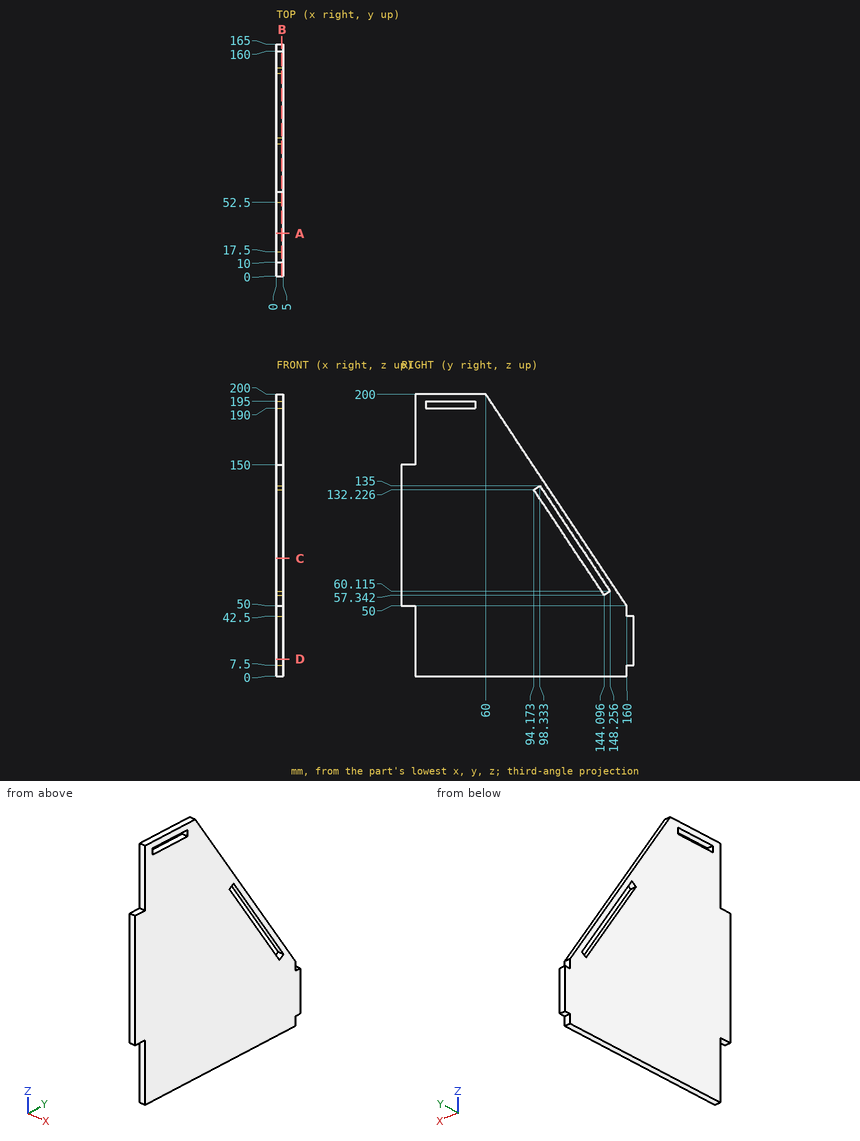
Study the drawing (mm; zero at the part's minimum x, y, z) and answer. Coordinates: 2 decimals unless noted, no trailing zeros. Order: outer loops, then holes, each group sorted by start corner. A loop starts at its lowest first (then second) coordinate and runs counter-clockwise, first axis right, second up. Notation, with made-up numbers: M -29,37.25 L -13,37.25 A25 ccw -13,55.25 Z; hole C -3,13 d9. An arc over 180 degrees is marked long. Use CSV: the item, a comma, the result in double quotes.
Q1. Section D-D (z = 12) is taken. Determine the outline of the cut face in (x, y), then the cut area to 3 significant figures.
Here are the results:
outline,"M 0,10 L 5,10 L 5,165 L 0,165 Z"
area,"775 mm2"
Q2. Section C-C (z = 83.5) is taken. Determine the outline of the cut face in (x, y).
Here are the results:
outline,"M 0,0 L 5,0 L 5,126.66 L 0,126.66 Z; M 0,132.67 L 5,132.67 L 5,137.67 L 0,137.67 Z"
Q3. Section A-A (y = 30.5) is taken. Determine the outline of the cut face in (x, z).
Here are the results:
outline,"M 0,0 L 5,0 L 5,190 L 0,190 Z; M 0,195 L 5,195 L 5,200 L 0,200 Z"
Q4. Straight lines are drawn through the part: L1, parallel to Z at x = 2.1, y = 45; L2, parallel to Y at x = 4.4, z = 47.5; L3, parallel to Y at x = 0.9, z = 32.5. For each, find the intervals that lie inside material, in ascending order.
Here are the results:
L1,"0 to 190, 195 to 200"
L2,"10 to 160"
L3,"10 to 165"
Q5. Section B-B (x = 3.9) is taken. Determine the outline of the cut face in (y, z) (1 decimal), then the cut area to 4 significant figures.
Here are the results:
outline,"M 0,50 L 10,50 L 10,0 L 160,0 L 160,7.5 L 165,7.5 L 165,42.5 L 160,42.5 L 160,50 L 60,200 L 10,200 L 10,150 L 0,150 Z; hole M 17.5,190 L 52.5,190 L 52.5,195 L 17.5,195 Z; hole M 94.2,132.2 L 144.1,57.3 L 148.3,60.1 L 98.3,135 Z"
area,"23,050 mm2"
Q6. Given pin 1 Ø2.5 at (x, z) = (2.5, 192.5) entering from -Y; pin 2 Ø1.5 at (x, z) = (3, 46) entering from +Y; pin 3 Ø3 at (x, z) = (2.5, 144) entering from +Y, each flat-ended and moving along its own axis, determine where each tip first touches the part or whether it passes through.
Here are the results:
pin 1,"y = 10"
pin 2,"y = 160"
pin 3,"y = 98.33"
